```python
from build123d import *

# Parameters (mm, degrees)
SKETCH_1_W          = 86
SKETCH_1_H          = 55
EXTRUDE_311_DEPTH   = 0.8
SKETCH_2_W          = 88
SKETCH_2_H          = 3.8
EXTRUDE_1_DEPTH     = 2
SKETCH_3_W          = 87.2
SKETCH_3_H          = 2.2
CUT_EXTRUDE_1_DEPTH = 1.4
SKETCH_4_W          = 59
SKETCH_4_H          = 3.8
EXTRUDE_2_DEPTH     = 2
SKETCH_5_W          = 57.8
SKETCH_5_H          = 2.2
CUT_EXTRUDE_2_DEPTH = 0.8


with BuildPart() as part:
    # Эскиз1 → Extrude 311 (new body)
    with BuildSketch(Plane(origin=(0, 0, 0), x_dir=(1, 0, 0), z_dir=(0, 1, 0))):
        Rectangle(SKETCH_1_W, SKETCH_1_H)
    extrude(amount=EXTRUDE_311_DEPTH)

    # Эскиз2 → Бобышка-Вытянуть1 (add)
    with BuildSketch(Plane(origin=(0, 0, -27.5), x_dir=(-1, 0, 0), z_dir=(0, 0, -1))):
        with Locations((1, 1.9)):
            Rectangle(SKETCH_2_W, SKETCH_2_H)
    extrude_1 = extrude(amount=EXTRUDE_1_DEPTH)

    # Эскиз3 → Вырез-Вытянуть1 (cut)
    with BuildSketch(Plane.XY.offset(-27.5)):
        with Locations((-0.6, 1.9)):
            Rectangle(SKETCH_3_W, SKETCH_3_H)
    cut_extrude_1 = extrude(amount=-CUT_EXTRUDE_1_DEPTH, mode=Mode.SUBTRACT)

    # Зеркальное отражение1: Бобышка-Вытянуть1, Вырез-Вытянуть1 across plane
    add(extrude_1.mirror(Plane.XY))
    add(cut_extrude_1.mirror(Plane.XY), mode=Mode.SUBTRACT)

    # Эскиз4 → Бобышка-Вытянуть2 (add)
    with BuildSketch(Plane.ZY.offset(43)):
        with Locations((0, 1.9)):
            Rectangle(SKETCH_4_W, SKETCH_4_H)
    extrude(amount=EXTRUDE_2_DEPTH)

    # Эскиз5 → Вырез-Вытянуть2 (cut)
    with BuildSketch(Plane(origin=(-43, 0, 0), x_dir=(0, 0, -1), z_dir=(1, 0, 0))):
        with Locations((0, 1.9)):
            Rectangle(SKETCH_5_W, SKETCH_5_H)
    extrude(amount=-CUT_EXTRUDE_2_DEPTH, mode=Mode.SUBTRACT)


solid = part.part
```
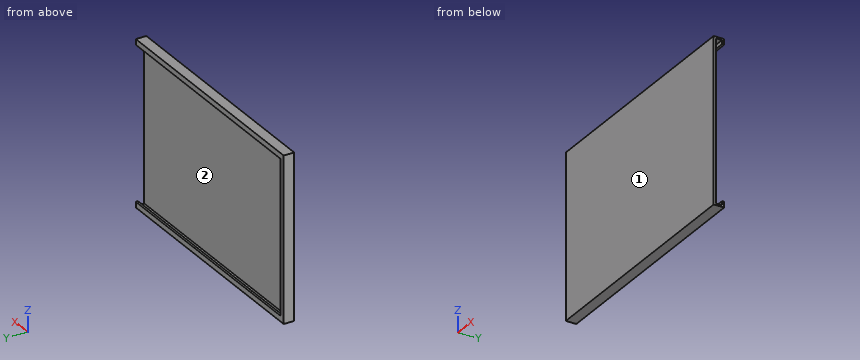
CAD build for the part. Positions are in the model's coordinates, mm. Face numbers are marked on the shaded views. Give positions to 0.01 mm unless a question says otherwise; leave off trailing zeros. Loops run counter-clockwise (first coordinate to the right, second up) from the corner with the lowest first, then second, coordinate; pieces in that order, holes last. Notation, with made-up numbers: (71, -14.5) - (118, -14.5) arc R14 cw to (118, -5.5) - close; hole circle Ø8 at (-4.5, 77). An arc over 180 degrees is marked (long way). Put each result on its own line as item: value.
Q1. Probe line 1 along Z through (x, y) = (2, 1.7); line 2 along Y through (x, z) = (19.5, 13.5); line 3 along Z through (x, y) = (11.5, 3.2). List the from-to ranges inside material, lowest first.
Filled in:
line 1: z = -29.5 to -28.9, 28.9 to 29.5
line 2: y = 0 to 0.8
line 3: z = -29.5 to -27.5, 27.5 to 29.5
Q2. Slice it at C-C (z = 19.5). Give the cut face in (x, y), plus the area to 3 significant figures.
Filled in:
outline: (-45, 0) - (43, 0) - (43, 0.8) - (-43.8, 0.8) - (-43.8, 3) - (-43, 3) - (-43, 3.8) - (-45, 3.8) - close
area: 74.6 mm²
Q3. Mould opens along Z. For the marked faces 1 and 2 say: pulls with the +Z half, pulls with the -Z half, needs draft (parallel to the pull), parting line crosses it, or undercut.
Filled in:
face 1: needs draft
face 2: undercut
Q4. Slice it at B-B (x = -22). Give the cut face in (y, z).
Filled in:
outline: (0, -29.5) - (3.8, -29.5) - (3.8, -27.5) - (3, -27.5) - (3, -28.9) - (0.8, -28.9) - (0.8, 28.9) - (3, 28.9) - (3, 27.5) - (3.8, 27.5) - (3.8, 29.5) - (0, 29.5) - close
Q5. Slice it at A-A (y = 2.4). Give the cut face in (x, z), plus the area to 3 significant figures.
Filled in:
outline: (-45, -29.5) - (43, -29.5) - (43, -28.9) - (-43.8, -28.9) - (-43.8, 28.9) - (43, 28.9) - (43, 29.5) - (-45, 29.5) - close
area: 175 mm²
Q6. Flat gauge pins, fed straight in: pin 1 (6 mm diameter, centred on x = -18.5, z = 5, fed in from +Y); pin 2 (0.6 mm diameter, centred on y = 3.5, z = -4, fed in from +X). Where does each tip first touch, or does it go through?
Filled in:
pin 1: stops at y = 0.8
pin 2: stops at x = -43
